Part model, mm, in its own coordinate system. A direction names the side the tool comes from. Coordinates: 2 decimals unless noted, no trailing zeros. Order: outer loops, then holes, each group sorted by start corner. A loop starts at its lowest first (then second) coordinate and runs counter-clockwise, first axis right, second up. Notation, with made-up numbers: (66, 71) - (122, 71) arc R25 cw to (122, 101) - close; hole circle Ø3 at (59.5, -3.75). An arc over 180 degrees is marked (long way). Use a Markdown table: item, result. Add a question column.
1) Saw through at A-A on y = 0. List the corners of the cut face in (x, z).
2) Drop flat-ended pins along their axis: P1, Ø2, axis at y = 2.5, z = 6.5, coming from the +X side; P2, Ø1.2, axis at x = -0.5, y = 0, coming from the +Z side; P3, Ø1.5, axis at x = 3, z = 8, coming from the +Y side. Give the stop position or say it passes through.
3) Tool access for faces 1 (the face through (0, 0, 6)), 2 (the face through (2, -2, 0)), 3 (the face through (0, 2, 18)): list every direction of +Z, -Z, +X, -X, +Y, -Y with a clear straight run to the whole face (end or side of a thin tool).
4) Wall check: L1, parallel to Y at x = 0, z = 19.85; L2, parallel to Z at x = -0.25, y = 1.25; L3, parallel to Y at x = -1.75, z = 4. Give the ranges that are in metal, low to high. Write a range as [from, to].
5) Two-plate mould, pull along X, no slides. Class faces 4 (the face through (0, 2, 3)), 5 (the face through (-0.867, 3.905, 10.357)), 6 (the face through (2, -2, 21)): +X half, -X half, draft (parallel to the pull), parting line (faces both ways), or undercut.
6) Saw through at D-D on z = 10. List the corners of the cut face in (x, y), then the cut area to 3 significant figures.
7) Saw through at C-C on z = 4.5. List the corners of the cut face in (x, y).
Autodesk Inventor part; units mm, degrees
ref_plane "YZ Plane" through (0, 0, 0) normal (1, 0, 0) x (0, 1, 0)
ref_plane "XZ Plane" through (0, 0, 0) normal (0, 1, 0) x (-1, 0, 0)
ref_plane "XY Plane" through (0, 0, 0) normal (0, 0, 1) x (1, 0, 0)
sketch "スケッチ1" plane through (0, 0, 0) normal (0, 0, 1) x (1, 0, 0)
  circle A0 centre (0, 0) radius 4
  circle A1 centre (0, 0) radius 2
  dimension "d0" = 8
  dimension "d1" = 4
extrude "押し出し1" add sketch "スケッチ1" along normal blind 21
fillet "フィレット1" radius 0.3 2 edges at (-4, 0, 21) (-4, 0, 0)
thread "ねじ1"
extrude "押し出し2" add sketch "スケッチ1" along normal blind 15 contours A1
extrude "押し出し3" cut sketch "スケッチ1" along normal blind 6 contours A1
thread "ねじ2"
properties part number "スペーサーM4L21アルミ" material "アルミニウム 2014-T4"
Results are:
| question | item | result |
|---|---|---|
| 1 | outline | (-4, 0.3) arc R0.3 ccw to (-3.7, 0) - (-2, 0) - (-2, 6) - (2, 6) - (2, 0) - (3.7, 0) arc R0.3 ccw to (4, 0.3) - (4, 20.7) arc R0.3 ccw to (3.7, 21) - (2, 21) - (2, 15) - (-2, 15) - (-2, 21) - (-3.7, 21) arc R0.3 ccw to (-4, 20.7) - close |
| 2 | P1 | x = 3.71 |
| 2 | P2 | z = 15 |
| 2 | P3 | y = 3.31 |
| 3 | face 1 | -Z |
| 3 | face 2 | -Z, +X, -X, +Y, -Y |
| 3 | face 3 | +Z |
| 4 | L1 | [-4, -2], [2, 4] |
| 4 | L2 | [6, 15] |
| 4 | L3 | [-3.6, -0.97], [0.97, 3.6] |
| 5 | face 4 | undercut |
| 5 | face 5 | parting line |
| 5 | face 6 | draft |
| 6 | outline | circle Ø8 at (0, 0) |
| 6 | area | 50.3 mm2 |
| 7 | outline | circle Ø8 at (0, 0); hole circle Ø4 at (0, 0) |
